Autodesk Inventor part; units mm, degrees
ref_plane "YZ Plane" through (0, 0, 0) normal (1, 0, 0) x (0, 1, 0)
ref_plane "XZ Plane" through (0, 0, 0) normal (0, 1, 0) x (-1, 0, 0)
ref_plane "XY Plane" through (0, 0, 0) normal (0, 0, 1) x (1, 0, 0)
sketch "Boceto1" plane through (0, 0, 0) normal (1, 0, 0) x (0, 1, 0)
  line L0 (0, 0) -> (25, 0)
  line L1 (25, 0) -> (25, -180)
  line L2 (25, -180) -> (0, -180)
  line L3 (0, -180) -> (0, 0)
  dimension "d0" = 25
  dimension "d1" = 180
extrude "Extrusión1" add sketch "Boceto1" along normal blind 3
sketch "Boceto2" plane through (3, 0, 0) normal (1, 0, 0) x (0, 0, -1)
  line L0 (180, 0) -> (180, 25)
  line L1 (180, 25) -> (0, 25)
  line L2 (0, 25) -> (0, 0)
  line L3 (0, 0) -> (180, 0)
  circle A0 centre (45, 12.5) radius 1.5875
  circle A1 centre (90, 12.5) radius 1.5875
  circle A2 centre (135, 12.5) radius 1.5875
  dimension "d4" = 3.175
  dimension "d5" = 45
  dimension "d8" = 45
  dimension "d15" = 45
extrude "Extrusión2" cut sketch "Boceto2" against normal blind 3 contours A0 | A1 | A2
properties part number "Pestaña"
Part model, mm, in its own coordinate system. Coordinates: 2 decimals unless noted, no trailing zeros. Order: outer loops, then holes, each group sorted by start corner. A loop starts at its lowest first (then second) coordinate and runs counter-clockwise, first axis right, second up.
(1) Probe L1, parallel to Y at x = 2, z = -45. List the from-to ranges inside material, lowest first.
Check sheet entries:
L1: y = 0 to 10.91, 14.09 to 25
(2) Slice it at A-A, the plane z = -45. Write the cut outline in (x, y), and give its area (3 significant figures).
Check sheet entries:
outline: (0, 0) - (3, 0) - (3, 10.91) - (0, 10.91) - close; (0, 14.09) - (3, 14.09) - (3, 25) - (0, 25) - close
area: 65.5 mm2
(3) Pull direction Z, two halves, no side cores. Call faces 1 (the face through (1, 0, -91)), 2 (the face through (1.521, 11.892, -46.466)), 3 (the face through (1, 13, -180)): pulls with the +Z half, pulls with the -Z half, needs draft (parallel to the pull), parting line crosses it, or undercut.
Check sheet entries:
face 1: needs draft
face 2: undercut
face 3: pulls with the -Z half
